```python
from build123d import *

# Parameters (mm, degrees)
SKETCH1_W           = 60
SKETCH1_H           = 250
BOSS_EXTRUDE1_DEPTH = 5
BOSS_EXTRUDE2_DEPTH = 27
SKETCH3_R           = 6
CUT_EXTRUDE1_DEPTH  = 146.773797371


with BuildPart() as part:
    # Sketch1 → Boss-Extrude1 (new body)
    with BuildSketch(Plane.XY):
        Rectangle(SKETCH1_W, SKETCH1_H)
    extrude(amount=BOSS_EXTRUDE1_DEPTH)

    # Sketch2 → Boss-Extrude2 (add)
    with BuildSketch(Plane(origin=(30, 0, 0), x_dir=(0, 0, -1), z_dir=(1, 0, 0))):
        with BuildLine():
            Line((-5, 125), (-5, 85))
            Line((-5, 85), (-25, 85))
            ThreePointArc((-25, 85), (-45, 105), (-25, 125))
            Line((-25, 125), (-5, 125))
        make_face()
    extrude(amount=-BOSS_EXTRUDE2_DEPTH)

    # Sketch3 → Cut-Extrude1 (cut, through all)
    with BuildSketch(Plane(origin=(30, 0, 0), x_dir=(0, 0, -1), z_dir=(1, 0, 0))):
        with Locations((-25, 105)):
            Circle(SKETCH3_R)
    extrude(amount=-CUT_EXTRUDE1_DEPTH, mode=Mode.SUBTRACT)


solid = part.part
```
CAD build for the part. Positions are in the model's coordinates, mm. A direction names the side the tool comes from. Give positions to 0.01 mm unless a question says otherwise; leave off trailing zeros. Order: outer loops, then holes, each group sorted by start corner. A loop starts at its lowest first (then second) coordinate and runs counter-clockwise, first axis right, second up.
(1) Saw through at C-C, the plane z = 22. Give the cut face in (x, y).
(2) Saw through at D-D, the plane y = -95.5. Give the cut face in (x, z), then the cut area to 3 significant figures.
(3) Tool access for faces 1 (the flat face through (17, 85, 15)), 2 (the flat face through (3, 101, 20)), 3 (the flat face through (13, 125, 10)): list every direction of +Z, -Z, +X, -X, +Y, -Y with a clear straight run to the whole face (end or side of a thin tool).
(4) Flat gauge pins, fed straight in: pin 1 (4 mm diameter, centred on x = -20, y = 94.5, fed in from +Z); pin 2 (20 mm diameter, centred on y = 101.5, z = 19.5, fed in from -X); pin 3 (10 mm diameter, centred on x = 17, z = 18, fed in from -Y). Where does each tip first touch, or does it go through?
(5) Drill centre lines: L1, parallel to Y at x = 17.75, z = 25; L2, parallel to Z at x = 11, y = -104.5; L3, parallel to X at y = 106, z = 14. Where is each one in solid material? Low to high.
(6) Saw through at A-A, the plane y = 105. Give the cut face in (x, z).
(7) Mould opens along Y. For faces 4 (the cylindrical face through (17, 105, 45)), 5 (the cylindrical face through (16.69, 110.95, 25.78)), 6 (the flat face through (0, -125, 2)) say: released by +Y, released by -Y, zero draft, split by the parting line, or undercut.
(8) Saw through at B-B, the plane x = 16. Give the cut face in (y, z).
Results found:
1. outline: (3, 85) - (30, 85) - (30, 99.8) - (3, 99.8) - close; (3, 110.2) - (30, 110.2) - (30, 125) - (3, 125) - close
2. outline: (-30, 0) - (30, 0) - (30, 5) - (-30, 5) - close
2. area: 300 mm2
3. face 1: +Z, +X, -X, -Y
3. face 2: +Z, -X, +Y, -Y
3. face 3: +Z, -Z, +X, -X, +Y
4. pin 1: stops at z = 5
4. pin 2: stops at x = 3
4. pin 3: stops at y = 85
5. L1: y = 85 to 99, 111 to 125
5. L2: z = 0 to 5
5. L3: x = 3 to 30
6. outline: (-30, 0) - (30, 0) - (30, 19) - (3, 19) - (3, 5) - (-30, 5) - close; (3, 31) - (30, 31) - (30, 45) - (3, 45) - close
7. face 4: split by the parting line
7. face 5: undercut
7. face 6: released by -Y
8. outline: (-125, 0) - (125, 0) - (125, 25) arc R20 ccw to (85, 25) - (85, 5) - (-125, 5) - close; hole circle Ø12 at (105, 25)
